from build123d import *

# Parameters (mm, degrees)
SKETCH4_R           = 6
BOSS_EXTRUDE2_DEPTH = 10


with BuildPart() as part:
    # Sketch1 → Revolve1 (revolve)
    with BuildSketch(Plane.XY):
        Polygon((18, 78), (20, 78), (20, 70), (0, 70), (-20, 70), (-20, 78), (-18, 78), (-18, 72), (0, 72), (18, 72), align=None)
    revolve(axis=Axis((0, 0, 0), (-1, 0, 0)))

    # Sketch2 → Revolve2 (revolve)
    with BuildSketch(Plane.XY):
        with BuildLine():
            Line((-20, 78), (20, 78))
            ThreePointArc((20, 78), (24.688711259, 98), (20, 118))
            ThreePointArc((20, 118), (0, 126.284271247), (-20, 118))
            ThreePointArc((-20, 118), (-24.688711259, 98), (-20, 78))
        make_face()
    revolve(axis=Axis((-54.573590753, 0, 0), (1, 0, 0)))

    # Sketch4 → Boss-Extrude2 (add)
    with BuildSketch(Plane.ZY.offset(20)):
        with BuildLine():
            Line((4.383711468, 8.987940463), (30.685980275, 62.915583241))
            ThreePointArc((30.685980275, 62.915583241), (41.14496766, 56.631189606), (50.353786024, 48.626085932))
            Line((50.353786024, 48.626085932), (7.193398003, 6.946583705))
            ThreePointArc((7.193398003, 6.946583705), (8.090169944, 5.877852523), (8.829475929, 4.694715628))
            Line((8.829475929, 4.694715628), (61.8063315, 32.863009395))
            ThreePointArc((61.8063315, 32.863009395), (66.573956141, 21.631189606), (69.318764812, 9.742117067))
            Line((69.318764812, 9.742117067), (9.902680687, 1.39173101))
            ThreePointArc((9.902680687, 1.39173101), (10, 0), (9.902680687, -1.39173101))
            Line((9.902680687, -1.39173101), (69.318764812, -9.742117067))
            ThreePointArc((69.318764812, -9.742117067), (66.573956141, -21.631189606), (61.8063315, -32.863009395))
            Line((61.8063315, -32.863009395), (8.829475929, -4.694715628))
            ThreePointArc((8.829475929, -4.694715628), (8.090169944, -5.877852523), (7.193398003, -6.946583705))
            Line((7.193398003, -6.946583705), (50.353786024, -48.626085932))
            ThreePointArc((50.353786024, -48.626085932), (41.14496766, -56.631189606), (30.685980275, -62.915583241))
            Line((30.685980275, -62.915583241), (4.383711468, -8.987940463))
            ThreePointArc((4.383711468, -8.987940463), (3.090169944, -9.510565163), (1.736481777, -9.84807753))
            Line((1.736481777, -9.84807753), (12.155372437, -68.936542711))
            ThreePointArc((12.155372437, -68.936542711), (0, -70), (-12.155372437, -68.936542711))
            Line((-12.155372437, -68.936542711), (-1.736481777, -9.84807753))
            ThreePointArc((-1.736481777, -9.84807753), (-3.090169944, -9.510565163), (-4.383711468, -8.987940463))
            Line((-4.383711468, -8.987940463), (-30.685980275, -62.915583241))
            ThreePointArc((-30.685980275, -62.915583241), (-41.14496766, -56.631189606), (-50.353786024, -48.626085932))
            Line((-50.353786024, -48.626085932), (-7.193398003, -6.946583705))
            ThreePointArc((-7.193398003, -6.946583705), (-8.090169944, -5.877852523), (-8.829475929, -4.694715628))
            Line((-8.829475929, -4.694715628), (-61.8063315, -32.863009395))
            ThreePointArc((-61.8063315, -32.863009395), (-66.573956141, -21.631189606), (-69.318764812, -9.742117067))
            Line((-69.318764812, -9.742117067), (-9.902680687, -1.39173101))
            ThreePointArc((-9.902680687, -1.39173101), (-10, 0), (-9.902680687, 1.39173101))
            Line((-9.902680687, 1.39173101), (-69.318764812, 9.742117067))
            ThreePointArc((-69.318764812, 9.742117067), (-66.573956141, 21.631189606), (-61.8063315, 32.863009395))
            Line((-61.8063315, 32.863009395), (-8.829475929, 4.694715628))
            ThreePointArc((-8.829475929, 4.694715628), (-8.090169944, 5.877852523), (-7.193398003, 6.946583705))
            Line((-7.193398003, 6.946583705), (-50.353786024, 48.626085932))
            ThreePointArc((-50.353786024, 48.626085932), (-41.14496766, 56.631189606), (-30.685980275, 62.915583241))
            Line((-30.685980275, 62.915583241), (-4.383711468, 8.987940463))
            ThreePointArc((-4.383711468, 8.987940463), (-3.090169944, 9.510565163), (-1.736481777, 9.84807753))
            Line((-1.736481777, 9.84807753), (-12.155372437, 68.936542711))
            ThreePointArc((-12.155372437, 68.936542711), (0, 70), (12.155372437, 68.936542711))
            Line((12.155372437, 68.936542711), (1.736481777, 9.84807753))
            ThreePointArc((1.736481777, 9.84807753), (3.090169944, 9.510565163), (4.383711468, 8.987940463))
        make_face()
        Circle(SKETCH4_R, mode=Mode.SUBTRACT)
    extrude(amount=-BOSS_EXTRUDE2_DEPTH)


solid = part.part
Geometry check sheet. Reference: the model listing, model coordinates, mm. A direction names the side the tool comes from. Give positions to 0.01 mm unless a question says otherwise; leave off trailing zeros. Write each loop counter-clockwise with the first axis right and the second up, starting at its lowest first coordinate (ties: lowest second). Pieces come first, ordered by that corner, then holes. Notation, with made-up numbers: M 9,64 L 63,64 A22 ccw 63,72 Z; hole C -15.5,22 d4. An arc over 180 degrees is marked long. One line per question, with ' | ' between items.
1. Set-up check for faces 1 (the face through (0.252, -10.154, 77.336)), 2 (the face through (-10, -15, 1)), 3 (the face through (-20, -16, 1)), 4 (the face through (-15.1, 28.1, 29.1)): record each of +Z, -Z, +X, -X, +Y, -Y from which the full face is reachable in a straight line by a thin tool's end or side.
Ans:
face 1: none | face 2: +X | face 3: -X | face 4: +X, -X
2. Scan lines: line 1 along Z through (x, y) = (-9, 0); line 2 along Z through (x, y) = (-5, 0); line 3 along Y through (x, z) = (-12, 63). Record each from-to range of solid material in increasing order. Write a range as from..to.
Ans:
line 1: -124.81..-78, -72..-70, 70..72, 78..124.81 | line 2: -125.84..-78, -72..-70, 70..72, 78..125.84 | line 3: -106.35..-45.99, -34.86..-8.85, 8.85..34.86, 45.99..106.35
3. Gauge pin test, flat ends, axial feed: pin 1 (1.5 mm diameter, centred on y = -79, z = -48, fed in from -X); pin 2 (3 mm diameter, centred on y = 91.5, z = 12, fed in from +X); pin 3 (10 mm diameter, centred on x = 3.5, z = -55, fed in from -Y). Record the tip position at first contact, or that the pin passes through.
Ans:
pin 1: x = -24.43 | pin 2: x = 24.49 | pin 3: y = -115.8
4. Cross-section at A-A (y = 14.5). Count the separate pieces of the cut face and the enclosed holes in it, plus the area to 3 significant figures.
Ans:
separate pieces: 5 | enclosed holes: 2 | area: 5,460 mm2
5. Cross-section at C-C (x = 11.5). Enter the section's corners in (y, z), plus the area to 3 significant figures.
Ans:
outline: C 0,0 d247.68; C 0,0 d144; hole C 0,0 d156; hole C 0,0 d140 | area: 30,000 mm2
